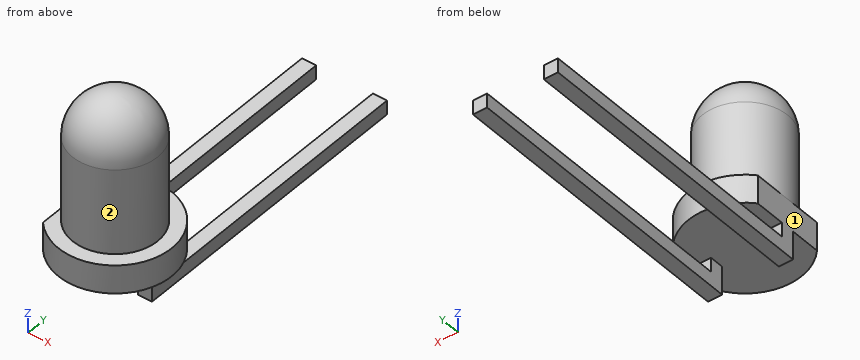
Autodesk Inventor part; units mm, degrees
ref_plane "YZ Plane" through (0, 0, 0) normal (1, 0, 0) x (0, 1, 0)
ref_plane "XZ Plane" through (0, 0, 0) normal (0, 1, 0) x (-1, 0, 0)
ref_plane "XY Plane" through (0, 0, 0) normal (0, 0, 1) x (1, 0, 0)
sketch "Skizze1" plane through (0, 0, 0) normal (0, 0, 1) x (1, 0, 0)
  circle A0 centre (0, 0) radius 1.5
  dimension "d0" = 3
extrude "Extrusion1" add sketch "Skizze1" along normal blind 5.5
fillet "Rundung1" radius 1.5 1 edges at (-1.5, 0, 5.5)
sketch "Skizze2" plane through (0, 0, 0) normal (0, 0, -1) x (-1, 0, 0)
  circle A0 centre (0, 0) radius 2
  line L0 (1.5, 1.3229) -> (1.5, -1.3229)
  circle A1 centre (0, 0) radius 1.5
  point P0 (1.5, 0)
  dimension "d4" = 4
extrude "Extrusion2" add sketch "Skizze2" against normal blind 1 contours L0 A0 picked at (-1.7994, 0.2793)
sketch "Skizze3" plane through (0, 0, 0) normal (0, 0, -1) x (-1, 0, 0)
  line L0 (1.5, -0.25) -> (1, -0.25)
  line L1 (1, -0.25) -> (1, 0.25)
  line L2 (1, 0.25) -> (1.5, 0.25)
  line L3 (1.5, 0.25) -> (1.5, -0.25)
  line L4 (-1, -0.25) -> (-1.5, -0.25)
  line L5 (-1.5, -0.25) -> (-1.5, 0.25)
  line L6 (-1.5, 0.25) -> (-1, 0.25)
  line L7 (-1, 0.25) -> (-1, -0.25)
  line L8 (1, 0) -> (-1, 0) construction
  point P0 (0, 0)
  point P1 (0, 0)
  point P2 (1.25, -0.25)
  point P3 (-1.25, -0.25)
  dimension "d7" = 0.5
  dimension "d9" = 2.5
extrude "Extrusion3" add sketch "Skizze3" along normal blind 1
sketch "Skizze4" plane through (-1.5, 0.25, 0) normal (0, 1, 0) x (1, 0, 0)
  line L0 (0, 0) -> (0, 1)
  line L1 (0.5, 0) -> (0.5, 1)
  line L2 (0, 1) -> (0.5, 1)
  line L3 (0.5, 1) -> (0.5, 0.5)
  line L4 (0.5, 0.5) -> (0, 0.5)
  line L5 (0, 0.5) -> (0, 1)
  line L6 (2.5, 0) -> (2.5, 1)
  line L7 (3, 0) -> (3, 1)
  line L8 (2.5, 1) -> (3, 1)
  line L9 (3, 1) -> (3, 0.5)
  line L10 (3, 0.5) -> (2.5, 0.5)
  line L11 (2.5, 0.5) -> (2.5, 1)
  point P0 (1.5, 0)
extrude "Extrusion4" add sketch "Skizze4" along normal blind 10
properties part number "LED 3mm" material "Silber"
Verification items for the finished model (mm, model axes). Face numbers are marked on the shaded views. A direction names the side the tool comes from. Give positions to 0.01 mm unless a question says otherwise; leave off trailing zeros. Write each loop counter-clockwise with the first axis right and the second up, starting at its lowest first coordinate (ties: lowest second). Pieces come first, ordered by that corner, then holes.
(1) Gauge pin test, flat ends, axial feed: pin 1 (0.5 mm diameter, centred on y = 5, z = -0.5, fed in from +X); pin 2 (2 mm diameter, centred on x = -1, z = 1.5, fed in from +Y). Record the tip position at first contact, or that the pin passes through.
(2) Material ranges on line 1 (Z direction, x = 0.95, y = 1.5); line 2 (Z direction, x = 1.25, y = 2.5); line 3 (X direction, y = 1, z = 4.5), recorded low to high.
(3) Cross-section at B-B (x = 0). Enter the section's corners in (y, z).
(4) Cross-section at C-C (z = 1.75). Enter the section's corners in (x, y).
(5) Cross-section at A-A (y = 6). Enter the section's corners in (x, z), plus the area to 3 significant figures.
(6) Access from +Z, -Z, +X, -X, +Y, -Y to the whole of each face (thin tool, end or side, straight path). Record for the marked faces 1 and 2.
(7) Cross-section at D-D (x = 1.3). Enter the section's corners in (y, z), plus the area to 3 significant figures.
Worked out:
1. pin 1: stops at x = 1.5
1. pin 2: stops at y = 2
2. line 1: z = 0 to 1
2. line 2: z = -1 to -0.5
2. line 3: x = -1 to 1
3. outline: (-2, 0) - (2, 0) - (2, 1) - (1.5, 1) - (1.5, 4) arc R1.5 ccw to (-1.5, 4) - (-1.5, 1) - (-2, 1) - close
4. outline: circle Ø3 at (0, 0)
5. outline: (-1.5, -1) - (-1, -1) - (-1, -0.5) - (-1.5, -0.5) - close; (1, -1) - (1.5, -1) - (1.5, -0.5) - (1, -0.5) - close
5. area: 0.500 mm2
6. face 1: +Z, -Z, -X, +Y, -Y
6. face 2: +Z
7. outline: (-1.52, 0) - (-0.25, 0) - (-0.25, -1) - (10.25, -1) - (10.25, -0.5) - (0.25, -0.5) - (0.25, 0) - (1.52, 0) - (1.52, 1) - (0.75, 1) - (0.75, 4) arc R0.75 ccw to (-0.75, 4) - (-0.75, 1) - (-1.52, 1) - close
7. area: 13.9 mm2
